Build history of the part. All positions in model axes, mm. Round coordinates to 2 decimals unless told otherwise and drop trailing zeros. Write each loop counter-clockwise with the first axis right and the second up, starting at its lowest first coordinate (ties: lowest second). Pieces come first, ordered by that corner, then holes.
Item 1: Drop a flat-ended pin along its axis: pin 1 Ø9 at (x, y) = (102.65, -57.66) entering from +Z. Give the stop position or say it passes through.
Item 2: Band-saw the part on C-C, the plane z = 3.3. Write the cut outline in (x, y).
Item 3: Mould opens along X. For faces 1 (the flat face through (56, -72.729, 2)), 2 (the cylindrical face through (107.607, -14.598, 2.465)), 3 (the cylindrical face through (112.88, -71.23, 2.54)), 4 (the cylindrical face through (2, -1, 3)) say: +X half, -X half, draft (parallel to the pull), parting line (faces both ways), or undercut.
Item 4: Wall check: probe 1 along X at (y, z) = (-13, 0.9); probe 2 along X at (y, z) = (-54.5, 2.2); probe 3 along Y at (x, z) = (10, 3.4). Give the ranges that are in metal, low to high.
Item 5: Band-saw the part on B-B, the plane x = 15. Write the cut outline in (y, z), then the cut area to 3 significant figures.
Item 6: Band-saw the part on A-A, the plane y = -61. Write the cut outline in (x, z).
```python
from build123d import *

# Parameters (mm, degrees)
F0_R     = 5.602125
F0_R_2   = 5.64379
F0_R_3   = 5.361194
F1_DEPTH = 5
F2_R     = 5
F3_R     = 5
F4_R     = 5
F5_R     = 5


with BuildPart() as f1:
    # F0 (on Top) → F1 (new body)
    with BuildSketch(Plane.XY):
        Polygon((57.153843, 0), (0, 0), (0, -72.72923), (114.307687, -72.72923), (114.307687, 0), align=None)
        with Locations((11.653123, -57.657372)):
            Circle(F0_R, mode=Mode.SUBTRACT)
        with Locations((102.654563, -57.657372)):
            Circle(F0_R, mode=Mode.SUBTRACT)
        with Locations((11.653123, -36.364615)):
            Circle(F0_R_2, mode=Mode.SUBTRACT)
        with Locations((11.653123, -12.544865)):
            Circle(F0_R_3, mode=Mode.SUBTRACT)
        with Locations((102.654563, -36.364615)):
            Circle(F0_R_2, mode=Mode.SUBTRACT)
        with Locations((102.654563, -12.544865)):
            Circle(F0_R_3, mode=Mode.SUBTRACT)
    extrude(amount=F1_DEPTH)

    # F2
    f2_edges = [f1.edges().sort_by_distance(p)[0] for p in [
        (114.307687, 0, 2.5),
    ]]
    fillet(f2_edges, radius=F2_R)

    # F3
    f3_edges = [f1.edges().sort_by_distance(p)[0] for p in [
        (0, 0, 2.5),
    ]]
    fillet(f3_edges, radius=F3_R)

    # F4
    f4_edges = [f1.edges().sort_by_distance(p)[0] for p in [
        (114.307687, -72.72923, 2.5),
    ]]
    fillet(f4_edges, radius=F4_R)

    # F5
    f5_edges = [f1.edges().sort_by_distance(p)[0] for p in [
        (0, -72.72923, 2.5),
    ]]
    fillet(f5_edges, radius=F5_R)


solid = f1.part
```
Results:
1. pin 1: passes through
2. outline: (0, -67.73) arc R5 ccw to (5, -72.73) - (109.31, -72.73) arc R5 ccw to (114.31, -67.73) - (114.31, -5) arc R5 ccw to (109.31, 0) - (5, 0) arc R5 ccw to (0, -5) - close; hole circle Ø11.29 at (11.65, -36.36); hole circle Ø11.2 at (11.65, -57.66); hole circle Ø10.72 at (11.65, -12.54); hole circle Ø11.29 at (102.65, -36.36); hole circle Ø11.2 at (102.65, -57.66); hole circle Ø10.72 at (102.65, -12.54)
3. face 1: draft
3. face 2: undercut
3. face 3: +X half
3. face 4: -X half
4. probe 1: x = 0 to 6.31, 16.99 to 97.31, 108 to 114.31
4. probe 2: x = 0 to 7.03, 16.28 to 98.03, 107.28 to 114.31
4. probe 3: y = -72.73 to -63.01, -52.3 to -41.76, -30.97 to -17.64, -7.44 to 0
5. outline: (-72.73, 0) - (-62.15, 0) - (-62.15, 5) - (-72.73, 5) - close; (-53.16, 0) - (-40.91, 0) - (-40.91, 5) - (-53.16, 5) - close; (-31.82, 0) - (-16.73, 0) - (-16.73, 5) - (-31.82, 5) - close; (-8.36, 0) - (0, 0) - (0, 5) - (-8.36, 5) - close
5. area: 231 mm2
6. outline: (0, 0) - (7.16, 0) - (7.16, 5) - (0, 5) - close; (16.15, 0) - (98.16, 0) - (98.16, 5) - (16.15, 5) - close; (107.15, 0) - (114.31, 0) - (114.31, 5) - (107.15, 5) - close
